Autodesk Inventor part; units mm, degrees
ref_plane "YZ Plane" through (0, 0, 0) normal (1, 0, 0) x (0, 1, 0)
ref_plane "XZ Plane" through (0, 0, 0) normal (0, 1, 0) x (-1, 0, 0)
ref_plane "XY Plane" through (0, 0, 0) normal (0, 0, 1) x (1, 0, 0)
sketch "Sketch1" plane through (0, 0, 0) normal (0, 0, 1) x (1, 0, 0)
  line L0 (9.7407, 1114.2593) -> (159.7407, 1114.2593)
  line L1 (9.7407, 1114.2593) -> (-140.2593, 1114.2593)
  line L2 (-943.4843, -492.1907) -> (-140.2593, 1114.2593)
  line L3 (159.7407, 1114.2593) -> (962.9657, -492.1907)
  line L4 (918.2444, -492.1907) -> (135.0194, 1074.2593)
  line L5 (135.0194, 1074.2593) -> (9.7407, 1074.2593)
  line L6 (9.7407, 1074.2593) -> (-115.5379, 1074.2593)
  line L7 (-115.5379, 1074.2593) -> (-898.7629, -492.1907)
  line L8 (9.7407, 554.2593) -> (395.0194, 554.2593)
  line L9 (9.7407, 554.2593) -> (-375.5379, 554.2593)
  line L10 (415.0194, 514.2593) -> (9.7407, 514.2593)
  line L11 (9.7407, 514.2593) -> (-395.5379, 514.2593)
  line L12 (-635.5379, 34.2593) -> (-680.2593, 34.2593)
  line L13 (9.7407, 34.2593) -> (9.7407, -477.7407)
  line L14 (-785.5379, -265.7407) -> (-830.2593, -265.7407)
  line L15 (-830.2593, -265.7407) -> (-785.5379, -265.7407)
  line L16 (911.0194, -477.7407) -> (955.7407, -477.7407)
  line L17 (955.7407, -477.7407) -> (911.0194, -477.7407)
  line L18 (-891.5379, -477.7407) -> (-936.2593, -477.7407)
  line L19 (918.2444, -492.1907) -> (962.9657, -492.1907)
  line L20 (-943.4843, -492.1907) -> (-898.7629, -492.1907)
  point P0 (0, 0)
  point P1 (655.0194, 34.2593)
  point P2 (699.7407, 34.2593)
  point P3 (-670.2593, 54.2593)
  dimension "d4" = 40
  dimension "d5" = 40
  dimension "d12" = 40
  dimension "d23" = 512
extrude "Extrusion1" add sketch "Sketch1" along normal blind 40 contours L0 L3 L16 L4 L5 L6 L7 L12 L2 L1
fillet "Fillet1" radius 0.5 7 edges at (-245.5379, 814.2593, 40) (-515.5379, 274.2593, 40) (72.3801, 1074.2593, 40) (265.0194, 814.2593, 40) (557.7407, 318.2593, 40) (-65.2593, 1114.2593, 40) (-410.2593, 574.2593, 40)
fillet "Fillet2" radius 0.5 7 edges at (-410.2593, 574.2593, 0) (-245.5379, 814.2593, 0) (-515.5379, 274.2593, 0) (72.3801, 1074.2593, 0) (84.7407, 1114.2593, 0) (557.7407, 318.2593, 0) (265.0194, 814.2593, 0)
extrude "Extrusion2" add sketch "Sketch1" along normal blind 40 contours L10 L11 L7 L9 L8 L4
fillet "Fillet3" radius 0.5 3 edges at (9.7407, 554.2593, 0) (212.3801, 514.2593, 0) (212.3801, 514.2593, 40)
fillet "Fillet4" radius 0.5 1 edges at (9.7407, 554.2593, 40)
sketch "Sketch2" plane through (-140.2593, 1114.2593, 39.5) normal (0, 1, 0) x (1, 0, 0)
  line L0 (298.84, 0.606) -> (0.309, 39.5)
  line L1 (299.691, 39.5) -> (0, 0)
  circle A0 centre (150.8669, 19.8846) radius 2.5
  point P0 (140.2593, 39.5)
  dimension "d17" = 5
extrude "Extrusion3" cut sketch "Sketch2" against normal blind 50
sketch "Sketch3" plane through (-140.2593, 1114.2593, 39.5) normal (0, 1, 0) x (1, 0, 0)
  point P0 (140.2593, 39.5)
sketch "Sketch4" plane through (-140.2593, 1114.2593, 39.5) normal (0, 1, 0) x (1, 0, 0)
  line L0 (226.7669, 24.5) -> (200.9669, 24.5)
  line L1 (226.7669, 24.5) -> (200.9669, 24.5)
  line L2 (200.9669, 14.5) -> (226.7669, 14.5)
  arc A0 (226.7669, 14.5) -> (226.7669, 24.5) centre (226.7669, 19.5) ccw
  arc A1 (200.9669, 24.5) -> (200.9669, 14.5) centre (200.9669, 19.5) ccw
  arc A2 (100.7669, 14.5) -> (100.7669, 24.5) centre (100.7669, 19.5) ccw
  line L3 (100.7669, 24.5) -> (74.9669, 24.5)
  line L4 (100.7669, 14.5) -> (74.9669, 14.5)
  arc A3 (74.9669, 24.5) -> (74.9669, 14.5) centre (74.9669, 19.5) ccw
  point P0 (140.2593, 39.5)
extrude "Extrusion4" cut sketch "Sketch4" against normal blind 50
extrude "Extrusion5" add sketch "Sketch1" along normal blind 40 contours L0 L3 L16 L4 L5 L6 L7 L12 L2 L1
extrude "Extrusion6" add sketch "Sketch1" along normal blind 40 contours L12 L7 L14 L2
extrude "Extrusion7" add sketch "Sketch1" along normal blind 40 contours L14 L7 L18 L2
extrude "Extrusion8" add sketch "Sketch1" along normal blind 40 contours L18 L7 L20 L2
extrude "Extrusion9" add sketch "Sketch1" along normal blind 40 contours L3 L19 L4 L16
sketch "Sketch5" plane through (-140.2593, 1114.2593, 0) normal (0, 1, 0) x (1, 0, 0)
  line L0 (535.5286, 0) -> (-235.5286, 0)
  line L1 (0.065, 0) -> (300, -40)
  line L2 (300, -40) -> (300, 0)
  line L3 (300, 0) -> (300, -40)
  line L4 (300, 0) -> (0.065, -40)
  circle A0 centre (150.0325, -20) radius 5
  point P0 (140.2593, 0)
  dimension "d38" = 10
extrude "Extrusion10" cut sketch "Sketch5" against normal blind 40 contours A0 L1 L4 | L4 L1 A0 | L1 L4 A0 | A0 L4 L1
sketch "Sketch6" plane through (-140.2593, 1114.2593, 0) normal (0, 1, 0) x (1, 0, 0)
  line L0 (225.9325, -25) -> (200.1325, -25)
  arc A0 (225.9325, -25) -> (225.9325, -15) centre (225.9325, -20) ccw
  line L1 (200.1325, -15) -> (225.9325, -15)
  arc A1 (200.1325, -15) -> (200.1325, -25) centre (200.1325, -20) ccw
  arc A2 (99.9325, -25) -> (99.9325, -15) centre (99.9325, -20) ccw
  line L2 (99.9325, -25) -> (74.1325, -25)
  arc A3 (74.1325, -15) -> (74.1325, -25) centre (74.1325, -20) ccw
  line L3 (74.1325, -15) -> (99.9325, -15)
  point P0 (140.2593, 0)
extrude "Extrusion11" cut sketch "Sketch6" against normal blind 50
properties part number "CAVALETE_SUPERIOR" material "SAE 1010/1020"
Work out the finished part from the listing and answer in its coordinate system (mm). A direction names the side the tool comes from. Give positions to 0.01 mm unless a question says otherwise; leave off trailing zeros. Write each loop counter-clockwise with the first axis right and the second up, starting at its lowest first coordinate (ties: lowest second). Pieces come first, ordered by that corner, then holes. Notation, with made-up numbers: (-24, -37.75) - (32, -37.75) arc R22 ccw to (32, -23.75) - close; hole circle Ø5 at (-24.5, 2.5). An arc over 180 degrees is marked (long way). Use one line per item in the form item = value.
1. A cutting plane is placed at A-A (z = 6.5). Write down the section's boundary in (x, y), and give its area (3 significant figures).
Filled in:
outline = (-943.48, -492.19) - (-898.76, -492.19) - (-395.54, 514.26) - (415.02, 514.26) - (918.24, -492.19) - (962.97, -492.19) - (159.74, 1114.26) - (-140.26, 1114.26) - close; hole (-375.54, 554.26) - (395.02, 554.26) - (135.02, 1074.26) - (-115.54, 1074.26) - close
area = 185,000 mm^2
2. For faces 4 (the face through (940, -492.191, 20)), 5 (the face through (-243.841, 817.653, 19.72)), 6 (the face through (-643.501, 18.333, 19.72)), determine the directions among +Z, -Z, +X, -X, +Y, -Y from which every point of the face is accessible in a straight line to the end or side of a thin tool.
Filled in:
face_4 = +Z, -Z, +X, -X, -Y
face_5 = +Z, -Z
face_6 = +Z, -Z, -Y
3. Determine the mould class of faces 1 (the face through (-921, -492.191, 20)), 2 (the face through (11, 1074.259, 11)), 3 (the face through (5, 553, 40)) for opening direction Y: released by +Y, released by -Y, zero draft, split by the parting line, or undercut.
Filled in:
face_1 = released by -Y
face_2 = undercut
face_3 = zero draft
4. Consider L1, parallel to X at y = 1103, z = 20; L2, parallel to X at y = 1088.5, z = 20; L3, parallel to X at y = 33.5, z = 37. Determine where each line is inside the solid, lowest interval first.
Filled in:
L1 = -145.89 to -71.13, -35.33 to 4.77, 14.77 to 54.87, 90.67 to 165.37
L2 = -153.14 to -71.13, -35.33 to 4.77, 14.77 to 54.87, 90.67 to 172.62
L3 = -680.64 to -635.92, 655.4 to 700.12
5. A cutting plane is placed at D-D (x = 843). Write down the section's boundary in (y, z), and give its area (3 significant figures).
Filled in:
outline = (-341.7, 0) - (-252.26, 0) - (-252.26, 40) - (-341.7, 40) - close
area = 3,580 mm^2
6. Each of these flat-tipped pins is pushed along its axis until it touches: pin 1 Ø12 at (x, z) = (13.5, 20) entering from -Y; pin 2 Ø4 at (x, z) = (452, 26) entering from -Y; pin 3 Ø1 at (y, z) = (688.5, 30.5) entering from +X. Where does it stop, or does it pass through?
Filled in:
pin_1 = 514.26
pin_2 = 436.3
pin_3 = 372.87
7. A cutting plane is placed at B-B (y = 834). Write down the section's boundary in (x, z).
Filled in:
outline = (-280.39, 0) - (-235.67, 0) - (-235.67, 40) - (-280.39, 40) - close; (255.15, 0) - (299.87, 0) - (299.87, 40) - (255.15, 40) - close
8. A cutting plane is placed at C-C (x = -277). Write down the section's boundary in (y, z).
Filled in:
outline = (514.26, 0.5) arc R0.5 ccw to (514.76, 0) - (553.76, 0) arc R0.5 ccw to (554.26, 0.5) - (554.26, 39.5) arc R0.5 ccw to (553.76, 40) - (514.76, 40) arc R0.5 ccw to (514.26, 39.5) - close; (751.34, 0) - (840.78, 0) - (840.78, 40) - (751.34, 40) - close
